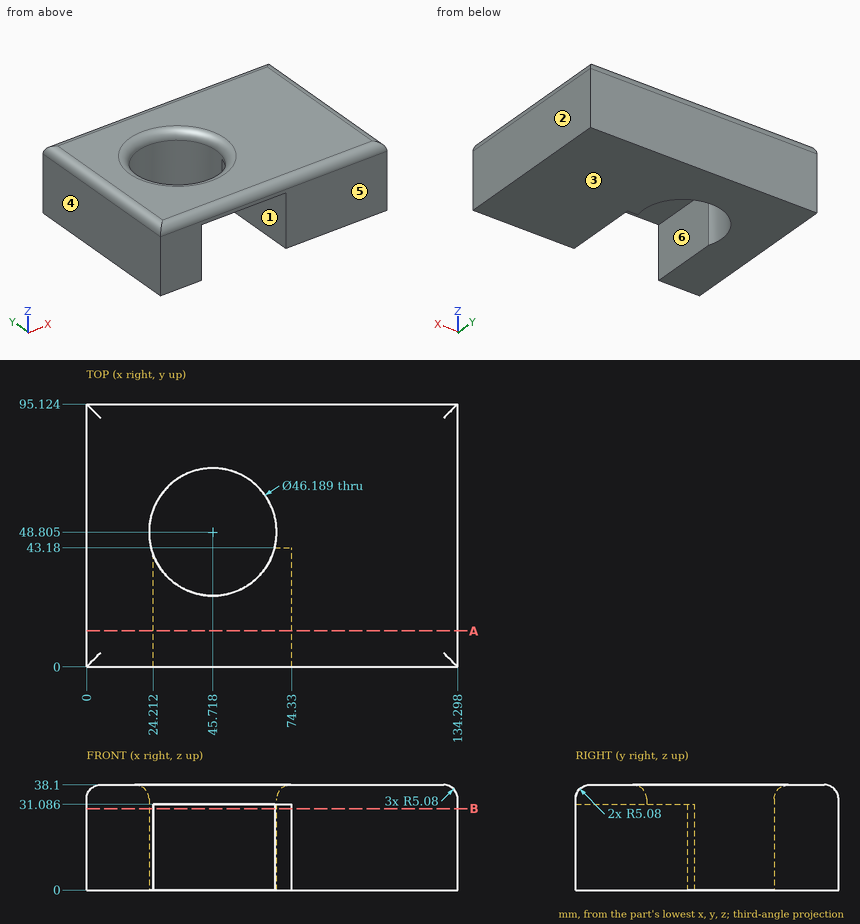
Source: three-view drawing plus pictorial views. Frame: mm from the lowest corner of the part. A direction names the side the tool comes from. Give positions to 0.01 mm unless a question says otherwise; leave off trailing zeros. Write each loop counter-clockwise with the first axis right and the second up, starting at its lowest first coordinate (ties: lowest second). Pieces come first, ordered by that corner, then holes. Notation, with made-up numbers: (74, -1) - (86, -1) arc R28 ccw to (86, 17) - close; hole circle Ø6 at (64, 45). An arc over 180 degrees is marked (long way). Write item = value, one per line. Start each with the question number.
1. Access query for the marked faces 5 and 6. Directions: +Z, -Z, +X, -X, +Y, -Y. A direction counts if a zero-diameter tool reaches every point of the face in a straight line with its end or side. Return the directions, or none.
2. Section query B-B, the plane z = 29.5. Output: boundary loops of the cut face in (x, y) (1 decimal).
3. Ray query, L1, parallel to X at y = 21, z = 4.5; L2, parallel to Z at x = 65, y = 5 (1 decimal); L3, parallel to X at y = 50, z = 5 (1 decimal). Return the intervals inside material, ascending.
4. Section query A-A, the plane y = 13. Output: boundary loops of the cut face in (x, z) (1 decimal).
5. First-contact query: pin 1 Ø3 at (x, z) = (71, 8.5) entering from -Y; pin 2 Ø21.5 at (x, y) = (54, 26.5) entering from -Z. Flat tips, straight axial feed; report the tip coordinate or a pass-through.
6. Mould query, pull axis X, two halves, no side actions, for the marked faces 1, 2, 3 and 4. Classes: released by +X, released by -X, zero draft, split by the parting line, or undercut.
Check sheet entries:
q1.face_5 = +Z, -Z, +X, -X, -Y
q1.face_6 = -Z, -Y
q2.outline = (0, 0) - (24.2, 0) - (24.2, 40.4) arc R23.1 cw (long way) to (68.1, 43.2) - (74.3, 43.2) - (74.3, 0) - (134.3, 0) - (134.3, 95.1) - (0, 95.1) - close
q3.L1 = 0 to 24.21, 74.33 to 134.3
q3.L2 = 31.1 to 38.1
q3.L3 = 0 to 22.7, 68.8 to 134.3
q4.outline = (0, 0) - (24.2, 0) - (24.2, 31.1) - (74.3, 31.1) - (74.3, 0) - (134.3, 0) - (134.3, 33) arc R5.1 ccw to (129.2, 38.1) - (5.1, 38.1) arc R5.1 ccw to (0, 33) - close
q5.pin_1 = 43.18
q5.pin_2 = 31.09
q6.face_1 = undercut
q6.face_2 = released by +X
q6.face_3 = zero draft
q6.face_4 = released by -X
